Geometry check sheet. Reference: the model listing, model coordinates, mm. A direction names the side the tool comes from. Give positions to 0.01 mm unless a question says otherwise; leave off trailing zeros. Order: outer loops, then holes, each group sorted by start corner. A loop starts at its lowest first (then second) coordinate and runs counter-clockwise, first axis right, second up. Notation, with made-up numbers: M 67.5,4 L 98.5,4 A8 ccw 98.5,12 Z; hole C 67.5,52 d6. An arc over 180 degrees is marked long. Answer as CSV lines item,"result".
from build123d import *

# Parameters (mm, degrees)
CROQUIS1_W                   = 55
CROQUIS1_H                   = 25
CROQUIS1_R                   = 2.75
SALIENTE_EXTRUIR1_DEPTH      = 2
SALIENTE_EXTRUIR1_DEPTH_BACK = 1.5
CROQUIS2_R                   = 4.75
CROQUIS2_R_2                 = 2.75
SALIENTE_EXTRUIR2_DEPTH      = 3.5
CROQUIS3_W                   = 55
CROQUIS3_H                   = 25
CROQUIS3_W_2                 = 51
CROQUIS3_H_2                 = 21
SALIENTE_EXTRUIR3_DEPTH      = 8
REDONDEO1_R                  = 3
CROQUIS5_W                   = 2
CROQUIS5_H                   = 11.102083366
CORTAR_EXTRUIR1_DEPTH        = 6
CROQUIS8_R                   = 4.5
CORTAR_EXTRUIR4_DEPTH        = 3
CROQUIS11_R                  = 2.75
SALIENTE_EXTRUIR5_DEPTH      = 5.5
CROQUIS12_R                  = 1.9
CORTAR_EXTRUIR11_DEPTH       = 9
CORTAR_EXTRUIR11_DEPTH_BACK  = 4.5
CROQUIS13_R                  = 2.5
CORTAR_EXTRUIR12_DEPTH       = 4.5
CROQUIS14_W                  = 1.5
CROQUIS14_H                  = 11.102083366
SALIENTE_EXTRUIR6_DEPTH      = 2


with BuildPart() as part:
    # Croquis1 → Saliente-Extruir1 (new body, two sides)
    with BuildSketch(Plane.XY) as saliente_extruir1_sk:
        Rectangle(CROQUIS1_W, CROQUIS1_H)
        with Locations((-10, 0)):
            Circle(CROQUIS1_R, mode=Mode.SUBTRACT)
        with Locations((11.5, 0)):
            Circle(CROQUIS1_R, mode=Mode.SUBTRACT)
    extrude(amount=SALIENTE_EXTRUIR1_DEPTH)
    extrude(saliente_extruir1_sk.sketch, amount=-SALIENTE_EXTRUIR1_DEPTH_BACK)

    # Croquis2 → Saliente-Extruir2 (add)
    with BuildSketch(Plane.XY.offset(2)):
        with Locations((-10, 0)):
            Circle(CROQUIS2_R)
        with Locations((-10, 0)):
            Circle(CROQUIS2_R_2, mode=Mode.SUBTRACT)
        with Locations((11.5, 0)):
            Circle(CROQUIS2_R)
        with Locations((11.5, 0)):
            Circle(CROQUIS2_R_2, mode=Mode.SUBTRACT)
    extrude(amount=SALIENTE_EXTRUIR2_DEPTH)

    # Croquis3 → Saliente-Extruir3 (add)
    with BuildSketch(Plane.XY.offset(2)):
        Rectangle(CROQUIS3_W, CROQUIS3_H)
        Rectangle(CROQUIS3_W_2, CROQUIS3_H_2, mode=Mode.SUBTRACT)
    extrude(amount=SALIENTE_EXTRUIR3_DEPTH)

    # Redondeo1
    redondeo1_edges = [part.edges().sort_by_distance(p)[0] for p in [
        (27.5, -12.5, 4.25),
        (-27.5, -12.5, 4.25),
        (-27.5, 12.5, 4.25),
        (27.5, 12.5, 4.25),
    ]]
    fillet(redondeo1_edges, radius=REDONDEO1_R)

    # Croquis5 → Cortar-Extruir1 (cut)
    with BuildSketch(Plane.XY.offset(10)):
        with Locations((26.5, 0)):
            Rectangle(CROQUIS5_W, CROQUIS5_H)
    extrude(amount=-CORTAR_EXTRUIR1_DEPTH, mode=Mode.SUBTRACT)

    # Croquis8 → Cortar-Extruir4 (cut)
    with BuildSketch(Plane.XY.offset(2)):
        with Locations((0.75, 0)):
            Circle(CROQUIS8_R)
        with Locations((-20.5, 0)):
            Circle(CROQUIS8_R)
        with Locations((20.501890269, 0)):
            Circle(CROQUIS8_R)
    extrude(amount=-CORTAR_EXTRUIR4_DEPTH, mode=Mode.SUBTRACT)

    # Croquis11 → Saliente-Extruir5 (add)
    with BuildSketch(Plane(origin=(0, 0, -1.5), x_dir=(-1, 0, 0), z_dir=(0, 0, -1))):
        with Locations((-11.5, 0)):
            Circle(CROQUIS11_R)
        with Locations((10, 0)):
            Circle(CROQUIS11_R)
    extrude(amount=-SALIENTE_EXTRUIR5_DEPTH)

    # Croquis12 → Cortar-Extruir11 (cut, two sides)
    with BuildSketch(Plane.XY.offset(2)) as cortar_extruir11_sk:
        with Locations((-10, 0)):
            Circle(CROQUIS12_R)
        with Locations((11.5, 0)):
            Circle(CROQUIS12_R)
    extrude(amount=CORTAR_EXTRUIR11_DEPTH, mode=Mode.SUBTRACT)
    extrude(cortar_extruir11_sk.sketch, amount=-CORTAR_EXTRUIR11_DEPTH_BACK, mode=Mode.SUBTRACT)

    # Croquis13 → Cortar-Extruir12 (cut, through all)
    with BuildSketch(Plane.XY.offset(2)):
        with Locations((20.501890269, 0)):
            Circle(CROQUIS13_R)
        with Locations((0.75, 0)):
            Circle(CROQUIS13_R)
        with Locations((-20.5, 0)):
            Circle(CROQUIS13_R)
    extrude(amount=-CORTAR_EXTRUIR12_DEPTH, mode=Mode.SUBTRACT)

    # Croquis14 → Saliente-Extruir6 (add)
    with BuildSketch(Plane(origin=(27.5, 0, 0), x_dir=(0, 0, -1), z_dir=(1, 0, 0))):
        with Locations((-4.75, 0)):
            Rectangle(CROQUIS14_W, CROQUIS14_H)
    extrude(amount=-SALIENTE_EXTRUIR6_DEPTH)


solid = part.part
(1) Tool access check on faces 4 (the face through (3, -2, -1)), 5 (the face through (-26.64, -11.6, 4.33)), 6 (the face through (-7, 0, 5.5)). Record the directions out of +Z, -Z, +X, -X, +Y, -Y that give a thin tool (end or side, any length) a straight path to the whole face; none if there is none.
The answers:
face 4,"+Z"
face 5,"+Z, -Z, -X, -Y"
face 6,"+Z, +X"
(2) Material ranges on line 1 (Y direction, x = 23.5, z = 4); line 2 (Y direction, x = 11.5, z = 2.6); line 3 (Y direction, x = 0.75, z = 0.1), recorded low to high.
The answers:
line 1,"y = -12.5 to -10.5, 10.5 to 12.5"
line 2,"y = -12.5 to -10.5, -4.75 to -1.9, 1.9 to 4.75, 10.5 to 12.5"
line 3,"y = -12.5 to -4.5, 4.5 to 12.5"
(3) Draft check along Y on faces 1 (the face through (0, 3, -1.5)), 2 (the face through (0, -12.5, 4)), 3 (the face through (-25, 0, 1)). Enter one of: +Y half, -Y half, draft (parallel to the pull), parting line (faces both ways), or undercut.
The answers:
face 1,"draft"
face 2,"-Y half"
face 3,"undercut"
(4) Section check B-B on x = -10. Enter the section's corners in (y, z).
The answers:
outline,"M -12.5,-1.5 L -1.9,-1.5 L -1.9,4 L -2.75,4 L -2.75,5.5 L -4.75,5.5 L -4.75,2 L -10.5,2 L -10.5,10 L -12.5,10 Z; M 1.9,-1.5 L 12.5,-1.5 L 12.5,10 L 10.5,10 L 10.5,2 L 4.75,2 L 4.75,5.5 L 2.75,5.5 L 2.75,4 L 1.9,4 Z"
(5) Gauge pin test, flat ends, axial feed: P1, Ø2.5, axis at x = -20, y = -1, coming from the +Z side; P2, Ø4.5, axis at x = 12.5, y = 0.5, coming from the +Z side; P3, Ø6.5, axis at x = -20.5, y = 0, coming from the +Z side; P4, Ø1.5, axis at x = -4, y = 2, coming from the +Z side. Record the tip position at first contact, or that the pin passes through.
The answers:
P1,"passes through"
P2,"stops at z = 5.5"
P3,"stops at z = -1"
P4,"stops at z = 2"
(6) Section check A-A on z = 2.75. Enter the section's corners in (x, y), then the cut area to 3 significant figures.
The answers:
outline,"M -27.5,-9.5 A3 ccw -24.5,-12.5 L 24.5,-12.5 A3 ccw 27.5,-9.5 L 27.5,9.5 A3 ccw 24.5,12.5 L -24.5,12.5 A3 ccw -27.5,9.5 Z; C -10,0 d9.5; C 11.5,0 d9.5; hole M -25.5,-10.5 L 25.5,-10.5 L 25.5,10.5 L -25.5,10.5 Z; hole C -10,0 d3.8; hole C 11.5,0 d3.8"
area,"415 mm2"
(7) Section check C-C on y = 8.75. Enter the section's corners in (x, z), then the cut area to 4 significant figures.
The answers:
outline,"M -27.5,-1.5 L 27.5,-1.5 L 27.5,10 L 25.5,10 L 25.5,2 L -25.5,2 L -25.5,10 L -27.5,10 Z"
area,"224.5 mm2"
(8) Section check D-D on x = -20.5. Enter the section's corners in (y, z), then the cut area to 3 significant figures.
The answers:
outline,"M -12.5,-1.5 L -2.5,-1.5 L -2.5,-1 L -4.5,-1 L -4.5,2 L -10.5,2 L -10.5,10 L -12.5,10 Z; M 2.5,-1.5 L 12.5,-1.5 L 12.5,10 L 10.5,10 L 10.5,2 L 4.5,2 L 4.5,-1 L 2.5,-1 Z"
area,"90.0 mm2"
